```python
from build123d import *

# Parameters (mm, degrees)
THICKEN1_T2   = 0.5
CHAMFER1_SIZE = 0.02
CHAMFER2_SIZE = 0.02


with BuildPart() as body_1:
    # Surface-Revolve1: a surface, the sketch's curves turned about an axis
    with BuildLine(Plane.XY, mode=Mode.PRIVATE) as surface_revolve1_1_path:
        Line((-1, 0), (-1, 28))
        ThreePointArc((-1, 28), (-0.707106781, 28.707106781), (0, 29))
    surface_revolve1_1 = Shell.revolve(surface_revolve1_1_path.wire(), 360, Axis((0, 0, 0), (0, 1, 0)))
    add(Solid.thicken(surface_revolve1_1, -THICKEN1_T2))

    # Chamfer1
    chamfer1_edges = [body_1.edges().sort_by_distance(p)[0] for p in [
        (1, 0, 0),
    ]]
    chamfer(chamfer1_edges, length=CHAMFER1_SIZE)

    # Chamfer2
    chamfer2_edges = [body_1.edges().sort_by_distance(p)[0] for p in [
        (0.5, 0, 0),
    ]]
    chamfer(chamfer2_edges, length=CHAMFER2_SIZE)

    # Sketch4 → Revolve2 (revolve)
    with BuildSketch(Plane.XY, mode=Mode.PRIVATE) as revolve2_sk:
        with BuildLine():
            Line((-1, 28), (0, 28))
            Line((0, 28), (0, 29))
            ThreePointArc((0, 29), (-0.707106781, 28.707106781), (-1, 28))
        make_face()
    revolve(revolve2_sk.sketch.rotate(Axis((0, 0, 0), (0, 1, 0)), 90), axis=Axis((0, 0, 0), (0, 1, 0)))


solid = body_1.part
```
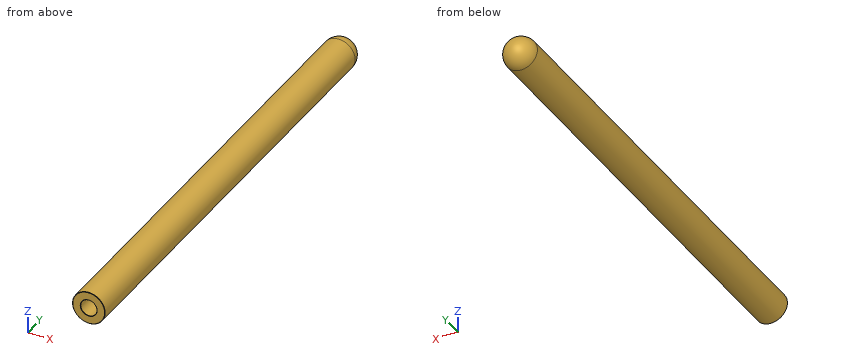
For this review, take the finished solid that the model builds, in its own axes (mm). Coordinates: 2 decimals unless noted, no trailing zeros. Write each loop counter-clockwise with the first axis right and the second up, starting at its lowest first coordinate (ties: lowest second). Pieces come first, ordered by that corner, then holes.
(1) Wall thickness on probe 1 along Z at (x, y) = (0, 20.5); probe 2 along Z at (x, y) = (0.3, 14): over which ranges is each line inside the solid? List them lowest first.
(2) For pin 1 Ø1 at (y, z) = (13, -1) entering from -X, flat-tipped, find the tip position at first contact; note if it passes through.
(3) Add section B-B on y = 3.5. Give the boundary of the cut face in (x, z), then the cut area to 3 significant figures.
Answer sheet:
1. probe 1: z = -1 to -0.5, 0.5 to 1
1. probe 2: z = -0.95 to -0.4, 0.4 to 0.95
2. pin 1: stops at x = -0.87
3. outline: circle Ø2 at (0, 0); hole circle Ø1 at (0, 0)
3. area: 2.36 mm2
